Verification items for the finished model (mm, model axes). Face numbers are marked on the shaded views. A direction names the side the tool comes from. Give positions to 0.01 mm unless a question says otherwise; leave off trailing zeros. Order: outer loops, then holes, each group sorted by start corner. A loop starts at its lowest first (then second) coordinate and runs counter-clockwise, first axis right, second up. Notation, with made-up numbers: (-2.75, 72.5) -> (16.25, 72.5) arc R31 cw to (16.25, 110.5) -> close; hole circle Ø1 at (24, 54.25). An arc over 180 degrees is marked (long way). Return JSON: item names as keys, results as strings. Group by question number.
(1) Cross-section at B-B on z = -8.5. Enter the section's corners in (x, y).
(2) Tool access check on the marked faces 5 and 6. Record the directions out of +Z, -Z, +X, -X, +Y, -Y that give a thin tool (end or side, any length) a straight path to the whole face; none if there is none.
(3) Cross-section at A-A on x = 113. Enter the section's corners in (y, z).
(4) Thickness scan on line 1 along X through (y, z) = (9.75, -10); line 2 along Z through (x, y) = (111, 6). Record the ranges inside material, lowest first.
(5) Release check for a two-part mould opening along Z. For the marked faces 1, 2, 3 and 4 record: pulls with the +Z half, pulls with the -Z half, needs draft (parallel to the pull), parting line crosses it, or undercut.
(6) Cross-section at C-C on y = 7.25. Enter the section's corners in (x, z).
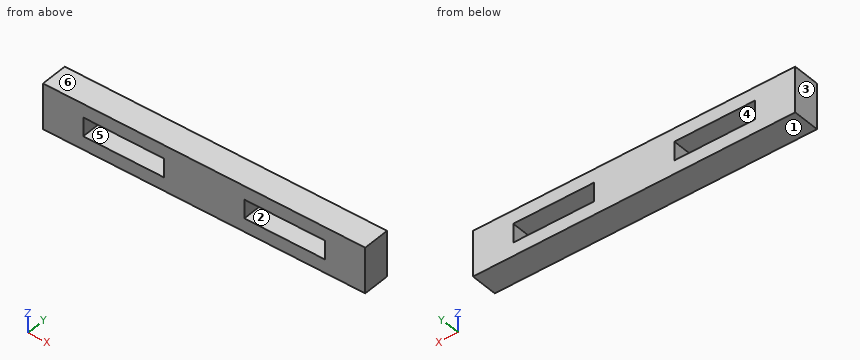
from build123d import *

# Parameters (mm, degrees)
SKETCH1_W               = 152.4
SKETCH1_H               = 21.59
BOSS_EXTRUDE1_DEPTH     = 12.7
SKETCH2_W               = 38.1
SKETCH2_H               = 8.89
CUT_EXTRUDE1_DEPTH      = 1
CUT_EXTRUDE1_DEPTH_BACK = 13.7


with BuildPart() as part:
    # Sketch1 → Boss-Extrude1 (new body)
    with BuildSketch(Plane(origin=(0, 0, 0), x_dir=(1, 0, 0), z_dir=(0, 1, 0))):
        with Locations((76.2, 10.795)):
            Rectangle(SKETCH1_W, SKETCH1_H)
    extrude(amount=BOSS_EXTRUDE1_DEPTH)

    # Sketch2 → Cut-Extrude1 (cut, two sides)
    with BuildSketch(Plane(origin=(0, 12.7, 0), x_dir=(1, 0, 0), z_dir=(0, 1, 0))) as cut_extrude1_sk:
        with Locations((38.1, 10.795)):
            Rectangle(SKETCH2_W, SKETCH2_H)
        with Locations((114.3, 10.795)):
            Rectangle(SKETCH2_W, SKETCH2_H)
    extrude(amount=CUT_EXTRUDE1_DEPTH, mode=Mode.SUBTRACT)
    extrude(cut_extrude1_sk.sketch, amount=-CUT_EXTRUDE1_DEPTH_BACK, mode=Mode.SUBTRACT)


solid = part.part
Verdict:
{
 "1": {"outline": "(0, 0) -> (19.05, 0) -> (19.05, 12.7) -> (0, 12.7) -> close; (57.15, 0) -> (95.25, 0) -> (95.25, 12.7) -> (57.15, 12.7) -> close; (133.35, 0) -> (152.4, 0) -> (152.4, 12.7) -> (133.35, 12.7) -> close"},
 "2": {"face 5": "+Y, -Y", "face 6": "+Z, +X, -X, +Y, -Y"},
 "3": {"outline": "(0, -21.59) -> (12.7, -21.59) -> (12.7, -15.24) -> (0, -15.24) -> close; (0, -6.35) -> (12.7, -6.35) -> (12.7, 0) -> (0, 0) -> close"},
 "4": {"line 1": "0 to 19.05, 57.15 to 95.25, 133.35 to 152.4", "line 2": "-21.59 to -15.24, -6.35 to 0"},
 "5": {"face 1": "pulls with the -Z half", "face 2": "undercut", "face 3": "needs draft", "face 4": "undercut"},
 "6": {"outline": "(0, -21.59) -> (152.4, -21.59) -> (152.4, 0) -> (0, 0) -> close; hole (19.05, -15.24) -> (57.15, -15.24) -> (57.15, -6.35) -> (19.05, -6.35) -> close; hole (95.25, -15.24) -> (133.35, -15.24) -> (133.35, -6.35) -> (95.25, -6.35) -> close"}
}
